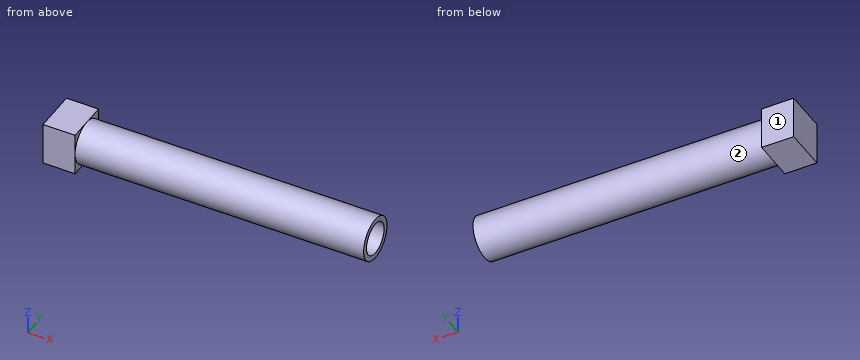
```python
from build123d import *

# Parameters (mm, degrees)
F0_W     = 20
F0_H     = 20
F1_DEPTH = 15
F2_R     = 10
F2_R_2   = 7.5
F3_DEPTH = 135


with BuildPart() as f1:
    # F0 (on Right) → F1 (new body)
    with BuildSketch(Plane.YZ):
        Rectangle(F0_W, F0_H)
    extrude(amount=F1_DEPTH)

    # F2 (on face) → F3 (join)
    with BuildSketch(Plane.YZ.offset(15)):
        Circle(F2_R)
        Circle(F2_R_2, mode=Mode.SUBTRACT)
    extrude(amount=F3_DEPTH)


solid = f1.part
```
The model under review builds one solid part; all positions refer to its coordinate system, in mm. Face numbers are marked on the shaded views. A direction names the side the tool comes from. Coordinates: 2 decimals unless noted, no trailing zeros. Write each loop counter-clockwise with the first axis right and the second up, starting at its lowest first coordinate (ties: lowest second). Pieces come first, ordered by that corner, then holes. Notation, with made-up numbers: (-17, 52.25) - (14, 52.25) arc R10 cw to (14, 58.25) - close; hole circle Ø4 at (51, 72.25). An arc over 180 degrees is marked (long way). Write item = value, one per line.
(1) Consider section A-A, the plane z = 6. Give the boundary of the cut face in (x, y).
Result sheet:
outline = (0, -10) - (15, -10) - (15, -8) - (150, -8) - (150, -4.5) - (15, -4.5) - (15, 4.5) - (150, 4.5) - (150, 8) - (15, 8) - (15, 10) - (0, 10) - close
(2) Machinability: for the marked faces 1 and 2, which of the approach directions +Z, -Z, +X, -X, +Y, -Y give a long, thin tool a straight path to every point of the face, cutting with its end or side? Answer none if there is none.
Result sheet:
face_1 = +Z, -Z, +X, -X, +Y
face_2 = +X
(3) For line 1 (Z direction, x = 85, y = 0); line 2 (X direction, y = 5, z = -1.25); line 3 (Y direction, x = 124, z = -2.75), list the stretches that pass through material, from the lowest coordinate up. Write a range as [from, to].
Result sheet:
line_1 = [-10, -7.5], [7.5, 10]
line_2 = [0, 15]
line_3 = [-9.61, -6.98], [6.98, 9.61]
(4) Consider section C-C, the plane x = 117. Give the boundary of the cut face in (y, z).
Result sheet:
outline = circle Ø20 at (0, 0); hole circle Ø15 at (0, 0)
(5) For P1, Ø12, axis at y = 0, z = 0, coming from the +X side; P2, Ø1, axis at x = 84, z = 7, coming from the +Y side; P3, Ø1, axis at x = 93, y = 5, coming from the -Z side, all flat-tipped, find the tip position at first contact; note any pin that passes through.
Result sheet:
P1 = 15
P2 = 7.6
P3 = -8.93
(6) Consider section B-B, the plane y = 1.5. Give the boundary of the cut face in (x, z), then the cut area to 3 significant figures.
Result sheet:
outline = (0, -10) - (15, -10) - (15, -9.89) - (150, -9.89) - (150, -7.35) - (15, -7.35) - (15, 7.35) - (150, 7.35) - (150, 9.89) - (15, 9.89) - (15, 10) - (0, 10) - close
area = 985 mm^2
